from build123d import *

# Parameters (mm, degrees)
SKETCH1_R           = 15
BOSS_EXTRUDE1_DEPTH = 40
FILLET1_R           = 12
SKETCH2_R           = 2
BOSS_EXTRUDE2_DEPTH = 30


with BuildPart() as part:
    # Sketch1 → Boss-Extrude1 (new body)
    with BuildSketch(Plane(origin=(0, 0, 0), x_dir=(1, 0, 0), z_dir=(0, 1, 0))):
        with Locations(Location((0, 0, 0), (0, 0, 270))):
            Circle(SKETCH1_R)
    extrude(amount=BOSS_EXTRUDE1_DEPTH)

    # Fillet1
    fillet1_edges = [part.edges().sort_by_distance(p)[0] for p in [
        (0, 0, -15),
        (0, 40, -15),
    ]]
    fillet(fillet1_edges, radius=FILLET1_R)

    # Sketch2 → Boss-Extrude2 (add)
    with BuildSketch(Plane(origin=(0, 40, 0), x_dir=(1, 0, 0), z_dir=(0, 1, 0))):
        with Locations(Location((0, 0, 0), (0, 0, 270))):
            Circle(SKETCH2_R)
    extrude(amount=BOSS_EXTRUDE2_DEPTH)


solid = part.part
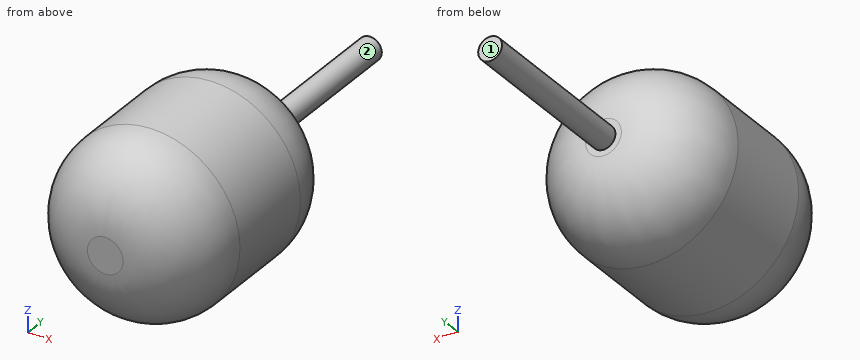
Here's how the part is built. I have some questions about the finished solid (model axes, mm). Face numbers are marked on the shaded views. A direction names the side the tool comes from. Coordinates: 2 decimals unless noted, no trailing zeros. Order: outer loops, then holes, each group sorted by start corner. A loop starts at its lowest first (then second) coordinate and runs counter-clockwise, first axis right, second up. Notation, with made-up numbers: M -15.5,80.25 L 14.5,80.25 A7 cw 14.5,87.25 Z; hole C 30,33 d2. An arc over 180 degrees is marked long. Answer as CSV lines item,"result". Start each with the question number.
1. I need wall thicknesses on line 1 (Y direction, x = -10.75, z = 8.25); line 2 (Z direction, x = -4, y = 27.5); line 3 (X direction, y = 14, z = -2). Which ranges of each line are inside material? Lowest first, please. Write a range as [from, to].
2. For pin 1 (4 mm diameter, centred on x = 11.5, z = -3, fed in from +Y); pin 2 (10 mm diameter, centred on x = 1, y = 21, fed in from -Z); pin 3 (10 mm diameter, centred on y = 59.5, z = -1, fed in from -X); pin 4 (4 mm diameter, centred on x = 11, z = 11.5, fed in from -Y), each with a flat end and sliding along its axis, tell me the tip position at first contact or that it passes through.
3. I want a section at A-A, the plane y = 54. Write out the boundary of the cut face in (x, z).
4. I want a section at B-B, the plane y = 23.5. Write out the boundary of the cut face in (x, z), and give its area (3 significant figures).
5. On a 3-axis mill with a long thin cutter (end or side, diameter ignored), from which of +Z, -Z, +X, -X, +Y, -Y can I reach the whole of each face in a straight line? I mean the marked faces 1 and 2. Say none if no direction works.
Recorded:
1,line 1,"y = [6.28, 33.72]"
1,line 2,"z = [-14.46, 14.46]"
1,line 3,"x = [-14.87, 14.87]"
2,pin 1,"stops at y = 37.83"
2,pin 2,"stops at z = -15"
2,pin 3,"stops at x = -2"
2,pin 4,"stops at y = 7.01"
3,outline,"C 0,0 d4"
4,outline,"C 0,0 d30"
4,area,"707 mm2"
5,face 1,"+Z, -Z, +X, -X, +Y"
5,face 2,"+Y"
